Can you work these out from the model? Positions are in its coordinate system, mm. Round coordinates to 2 decimals unless told otherwise and drop trailing zeros. Order: outer loops, then holes, each group sorted by start corner. A loop starts at its lowest first (then second) coordinate and runs counter-clockwise, first axis right, second up.
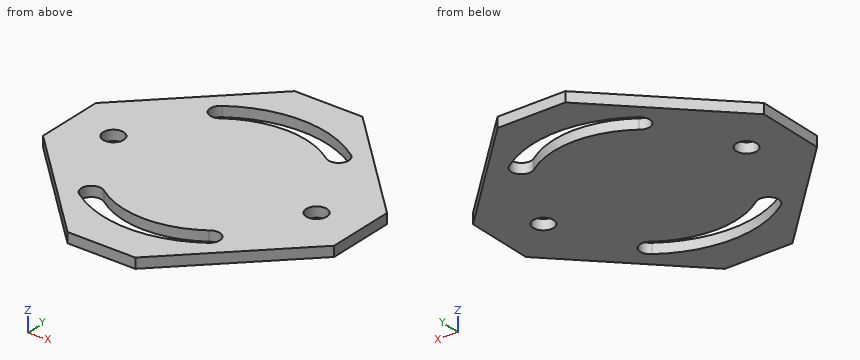
from build123d import *

# Parameters (mm, degrees)
SKETCH_1_R      = 3.0499512
EXTRUDE_1_DEPTH = 3


with BuildPart() as part:
    # 草图1 → 凸台-拉伸1 (new body)
    with BuildSketch(Plane.XY):
        Polygon((43.039042287, -10.445300798), (43.039042287, 9.554379202), (10.039570287, 42.553851202), (-9.960109713, 42.553851202), (-42.959581713, 9.554379202), (-42.959581713, -10.445300798), (-9.960109713, -43.444772798), (10.039570287, -43.444772798), align=None)
        with Locations((30.039250287, -0.445460798)):
            Circle(SKETCH_1_R, mode=Mode.SUBTRACT)
        with Locations((-29.959789713, -0.445460798)):
            Circle(SKETCH_1_R, mode=Mode.SUBTRACT)
        with BuildLine():
            ThreePointArc((15.536857472, 21.66371651), (0.039730287, 26.554107202), (-15.457396897, 21.66371651))
            ThreePointArc((-15.457396897, 21.66371651), (-19.856993747, 22.224541332), (-18.924411805, 26.56058421))
            ThreePointArc((-18.924411805, 26.56058421), (0.039730287, 32.554011202), (19.00387238, 26.56058421))
            ThreePointArc((19.00387238, 26.56058421), (19.936454322, 22.224541332), (15.536857472, 21.66371651))
        make_face(mode=Mode.SUBTRACT)
        with BuildLine():
            ThreePointArc((-15.457396897, -22.554638105), (0.039730287, -27.445028798), (15.536857472, -22.554638105))
            ThreePointArc((15.536857472, -22.554638105), (19.936454322, -23.115462927), (19.00387238, -27.451505806))
            ThreePointArc((19.00387238, -27.451505806), (0.039730287, -33.444932798), (-18.924411805, -27.451505806))
            ThreePointArc((-18.924411805, -27.451505806), (-19.856993747, -23.115462927), (-15.457396897, -22.554638105))
        make_face(mode=Mode.SUBTRACT)
    extrude(amount=EXTRUDE_1_DEPTH)


solid = part.part
(1) Please list where these lines run through material, in increasing order: probe 1 along Y at (x, z) = (-13, 0.65); probe 2 along Y at (x, z) = (19, 1.55); probe 3 along X at (y, z) = (-31, 0.85).
(2) I want a section at A-A, the plane y = 25. List the corners of the cut face in (x, z) for me, plus the area to 3 significant figures.
(3) I want a section at B-B, the plane x = 5. List the corners of the cut face in (y, z) for me, plus the area to 3 significant figures.
(4) I want a section at D-D, the plane z = 0.5. List the corners of the cut face in (x, y) for me, plus the area to 3 significant figures.
(5) I want a section at C-C, the plane y = -31. List the corners of the cut face in (x, z) for me, plus the area to 3 significant figures.
Ans:
1. probe 1: y = -40.4 to -30.76, -24.09 to 23.2, 29.87 to 39.51
1. probe 2: y = -34.48 to -27.45, -22.26 to 21.37, 26.56 to 33.59
1. probe 3: x = -22.4 to -12.43, 12.51 to 22.48
2. outline: (-27.51, 0) - (-20.23, 0) - (-20.23, 3) - (-27.51, 3) - close; (-8.99, 0) - (9.07, 0) - (9.07, 3) - (-8.99, 3) - close; (20.31, 0) - (27.59, 0) - (27.59, 3) - (20.31, 3) - close
2. area: 97.9 mm2
3. outline: (-43.44, 0) - (-33.07, 0) - (-33.07, 3) - (-43.44, 3) - close; (-26.99, 0) - (26.09, 0) - (26.09, 3) - (-26.99, 3) - close; (32.18, 0) - (42.55, 0) - (42.55, 3) - (32.18, 3) - close
3. area: 221 mm2
4. outline: (-42.96, -10.45) - (-9.96, -43.44) - (10.04, -43.44) - (43.04, -10.45) - (43.04, 9.55) - (10.04, 42.55) - (-9.96, 42.55) - (-42.96, 9.55) - close; hole circle Ø6.1 at (-29.96, -0.45); hole (-18.92, -27.45) arc R33 ccw to (19, -27.45) arc R3.01 ccw (long way) to (15.54, -22.55) arc R27 cw to (-15.46, -22.55) arc R3.01 ccw (long way) to start; hole (-18.92, 26.56) arc R3.01 ccw (long way) to (-15.46, 21.66) arc R27 cw to (15.54, 21.66) arc R3.01 ccw (long way) to (19, 26.56) arc R33 ccw to start; hole circle Ø6.1 at (30.04, -0.45)
4. area: 4,660 mm2
5. outline: (-22.4, 0) - (-12.43, 0) - (-12.43, 3) - (-22.4, 3) - close; (12.51, 0) - (22.48, 0) - (22.48, 3) - (12.51, 3) - close
5. area: 59.9 mm2
